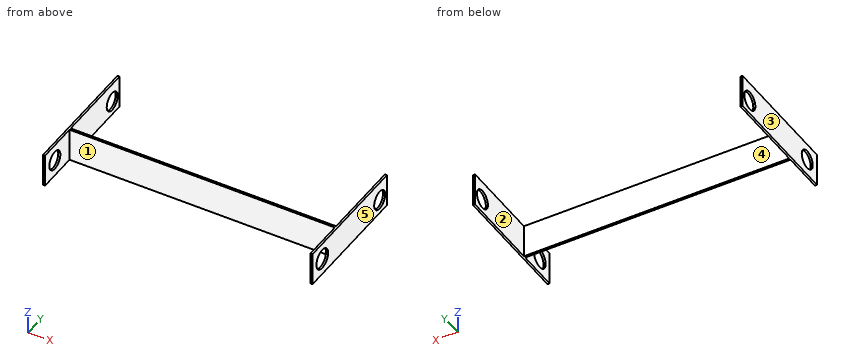
from build123d import *

# Parameters (mm, degrees)
BOSS_EXTRUDE1_DEPTH = 50.8
SKETCH3_W           = 50.8
SKETCH3_H           = 63.5
SKETCH3_R           = 14.2875
BOSS_EXTRUDE2_DEPTH = 3.175
SKETCH4_W           = 50.8
SKETCH4_H           = 63.5
SKETCH4_R           = 15.24
BOSS_EXTRUDE3_DEPTH = 3.175
SKETCH5_R           = 14.2875
CUT_EXTRUDE1_DEPTH  = 508


with BuildPart() as part:
    # Sketch2 → Boss-Extrude1 (new body)
    with BuildSketch(Plane.XY):
        Polygon((0, 0), (0, 130.175), (-3.175, 130.175), (-3.175, 3.175), (-409.575, 3.175), (-409.575, 130.175), (-412.75, 130.175), (-412.75, 0), align=None)
    extrude(amount=BOSS_EXTRUDE1_DEPTH)

    # Sketch3 → Boss-Extrude2 (add)
    with BuildSketch(Plane.ZY.offset(412.75)):
        with Locations((25.4, -31.75)):
            Rectangle(SKETCH3_W, SKETCH3_H)
        with Locations((25.4, -38.1)):
            Circle(SKETCH3_R, mode=Mode.SUBTRACT)
    extrude(amount=-BOSS_EXTRUDE2_DEPTH)

    # Sketch4 → Boss-Extrude3 (add)
    with BuildSketch(Plane(origin=(0, 0, 0), x_dir=(0, 0, -1), z_dir=(1, 0, 0))):
        with Locations((-25.4, -31.75)):
            Rectangle(SKETCH4_W, SKETCH4_H)
        with Locations((-25.4, -38.1)):
            Circle(SKETCH4_R, mode=Mode.SUBTRACT)
    extrude(amount=-BOSS_EXTRUDE3_DEPTH)

    # Sketch5 → Cut-Extrude1 (cut)
    with BuildSketch(Plane(origin=(0, 0, 0), x_dir=(0, 0, -1), z_dir=(1, 0, 0))):
        with Locations((-21.7297, 111.125)):
            Circle(SKETCH5_R)
    extrude(amount=-CUT_EXTRUDE1_DEPTH, mode=Mode.SUBTRACT)


solid = part.part
Geometry: final body of the model. Coordinates: model frame, mm. Face numbers are marked on the shaded views. A direction names the side the tool comes from. Give positions to 0.01 mm unless a question says otherwise; leave off trailing zeros. Loops run counter-clockwise (first coordinate to the right, second up) from the corner with the lowest first, then second, coordinate; pieces in that order, holes last. Notation, with made-up numbers: M 22.25,36.25 L 67.25,36.25 A14 cw 67.25,44.25 Z; hole C 6.5,-2.5 d9. An arc over 180 degrees is marked long. Put each result on its own line as item: value. Start each with the question number.
1) Contact query for flat-ended pins moving along their axis: pin 1 (10 mm diameter, centred on x = -363.5, z = 27, fed in from -Y); pin 2 (10 mm diameter, centred on x = -232, z = 9, fed in from +Y) (3 decimals); pin 3 (17 mm diameter, centred on y = -38.1, z = 25.4, fed in from -X). Output: stop coordinate, or through.
2) Cut plane D-D (x = -351.5). Output: boundary loops of the cut face in (y, z) (3 decimals).
3) Access query for the marked faces 1 and 2. Directions: +Z, -Z, +X, -X, +Y, -Y. A direction counts if a zero-diameter tool reaches every point of the face in a straight line with its end or side. Return the directions, or none.
4) Cut plane B-B (y = 31). Output: boundary loops of the cut face in (x, z) (3 decimals), then the cut area to 3 significant figures.
5) Ray query, line 1 along X through (y, z) = (98, 6.5) (3 decimals); line 2 along Y through (x, z) = (-1.8, 25.4) (3 decimals); line 3 along Y through (x, z) = (-197, 9.5) (3 decimals). Return the intervals inside material, ascending.
6) Cut plane A-A (y = -38.1). Give the number of separate pieces and of enclosed holes in the cut face, then the cut area to 3 significant figures.
7) Pull-direction query (X, two-part tool) for the marked faces 3, 4 and 5; classes: pulls with the +X half, pulls with the -X half, needs draft (parallel to the pull), parting line crosses it, or undercut.
Verdict:
1. pin 1: y = 0
1. pin 2: y = 3.175
1. pin 3: through
2. outline: M 0,0 L 3.175,0 L 3.175,50.8 L 0,50.8 Z
3. face 1: +Z, -Z, -Y
3. face 2: +Z, -Z, +Y
4. outline: M -412.75,0 L -409.575,0 L -409.575,50.8 L -412.75,50.8 Z; M -3.175,0 L 0,0 L 0,50.8 L -3.175,50.8 Z
4. area: 323 mm2
5. line 1: -412.75 to -409.575, -3.175 to 0
5. line 2: -63.5 to -53.34, -22.86 to 97.317, 124.933 to 130.175
5. line 3: 0 to 3.175
6. separate pieces: 4
6. enclosed holes: 0
6. area: 135 mm2
7. face 3: pulls with the -X half
7. face 4: undercut
7. face 5: pulls with the +X half
